from build123d import *

# Parameters (mm, degrees)
SKETCH158_R          = 1.85
PAD009_DEPTH         = 6
SKETCH159_R          = 5
PAD010_DEPTH         = 5
PAD010_DEPTH_BACK    = 6
SKETCH160_R          = 1.85
POCKET006_DEPTH      = 6.001
POCKET006_DEPTH_BACK = 5.001
POCKET007_DEPTH      = 3
SKETCH162_W          = 18
SKETCH162_H          = 8
PAD011_DEPTH         = 2
PAD011_DEPTH_BACK    = 9
PAD012_DEPTH         = 12
POCKET008_DEPTH      = 5
CHAMFER_SIZE         = 1


with BuildPart() as part:
    # Sketch158 → Pad009 (new body)
    with BuildSketch(Plane.XY):
        Polygon((-91, -102), (-91, 88), (0, 88), (0, 79), (-70, 79), (-81, 68), (-81, -64), (-70, -75), (0, -75), (0, -84), (-82, -84), (-82, -102), align=None)
        with Locations((-85, 84)):
            Circle(SKETCH158_R, mode=Mode.SUBTRACT)
        with Locations((-85, -7)):
            Circle(SKETCH158_R, mode=Mode.SUBTRACT)
        with Locations((-85, -98)):
            Circle(SKETCH158_R, mode=Mode.SUBTRACT)
        with Locations((-85, 43)):
            Circle(SKETCH158_R, mode=Mode.SUBTRACT)
        with Locations((-85, -37)):
            Circle(SKETCH158_R, mode=Mode.SUBTRACT)
    pad009 = extrude(amount=PAD009_DEPTH)

    # Mirrored: Pad009 across Sketch158 V_Axis
    add(pad009.mirror(Plane(origin=(0, 0, 0), x_dir=(0, 0, 1), z_dir=(1, 0, 0))))

    # Sketch159 → Pad010 (join, two sides)
    with BuildSketch(Plane.XY.offset(6)) as pad010_sk:
        with Locations((-79, 78)):
            Circle(SKETCH159_R)
        with Locations((-79, -76.94)):
            Circle(SKETCH159_R)
        with Locations((78.48, -76.94)):
            Circle(SKETCH159_R)
        with Locations((78.48, 55.14)):
            Circle(SKETCH159_R)
    extrude(amount=PAD010_DEPTH)
    extrude(pad010_sk.sketch, amount=-PAD010_DEPTH_BACK)

    # Sketch160 → Pocket006 (cut, two sides)
    with BuildSketch(Plane.XY.offset(6)) as pocket006_sk:
        with Locations((-79, 78)):
            Circle(SKETCH160_R)
        with Locations((-79, -76.94)):
            Circle(SKETCH160_R)
        with Locations((78.48, -76.94)):
            Circle(SKETCH160_R)
        with Locations((78.48, 55.14)):
            Circle(SKETCH160_R)
    extrude(amount=-POCKET006_DEPTH, mode=Mode.SUBTRACT)
    extrude(pocket006_sk.sketch, amount=POCKET006_DEPTH_BACK, mode=Mode.SUBTRACT)

    # Sketch161 → Pocket007 (cut)
    with BuildSketch(Plane.XY.offset(11)):
        Polygon((-75.709103, 78), (-77.354552, 80.85), (-80.645448, 80.85), (-82.290897, 78), (-80.645448, 75.15), (-77.354552, 75.15), align=None)
        Polygon((81.770897, 55.14), (80.125448, 57.99), (76.834552, 57.99), (75.189103, 55.14), (76.834552, 52.29), (80.125448, 52.29), align=None)
        Polygon((81.770897, -76.94), (80.125448, -74.09), (76.834552, -74.09), (75.189103, -76.94), (76.834552, -79.79), (80.125448, -79.79), align=None)
        Polygon((-75.709103, -76.94), (-77.354552, -74.09), (-80.645448, -74.09), (-82.290897, -76.94), (-80.645448, -79.79), (-77.354552, -79.79), align=None)
    extrude(amount=-POCKET007_DEPTH, mode=Mode.SUBTRACT)

    # Sketch162 → Pad011 (join, two sides)
    with BuildSketch(Plane(origin=(0, 88, 0), x_dir=(-1, 0, 0), z_dir=(0, 1, 0))) as pad011_sk:
        with Locations((67, 4)):
            Rectangle(SKETCH162_W, SKETCH162_H)
    extrude(amount=PAD011_DEPTH)
    extrude(pad011_sk.sketch, amount=-PAD011_DEPTH_BACK)

    # Sketch166 (on Face53 of Pad011) → Pad012 (join)
    with BuildSketch(Plane(origin=(0, 90, 0), x_dir=(-1, 0, 0), z_dir=(0, 1, 0))):
        Polygon((73, 0), (65, 0), (65, 116), (103, 116), (103, 111), (73, 111), align=None)
    extrude(amount=PAD012_DEPTH)

    # Sketch167 (on Face88 of Pad012) → Pocket008 (cut)
    with BuildSketch(Plane.XY.offset(116)):
        with BuildLine():
            ThreePointArc((-97.5, 98.5), (-100, 96), (-97.5, 93.5))
            Line((-97.5, 93.5), (-82.5, 93.5))
            ThreePointArc((-82.5, 93.5), (-80, 96), (-82.5, 98.5))
            Line((-97.5, 98.5), (-82.5, 98.5))
        make_face()
    extrude(amount=-POCKET008_DEPTH, mode=Mode.SUBTRACT)

    # Chamfer
    chamfer_edges = [part.edges().sort_by_distance(p)[0] for p in [
        (-69, 90, 8),
    ]]
    chamfer(chamfer_edges, length=CHAMFER_SIZE)


with BuildPart() as part_1:
    # Body006 placement: moved
    add(part.part.moved(Location((0, 2, 118))))


solid = part_1.part
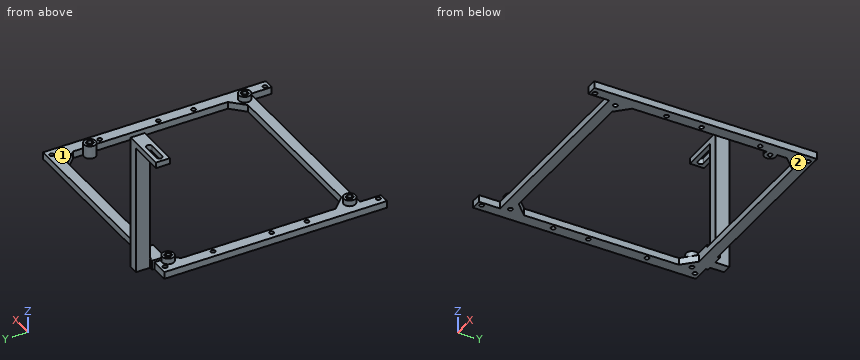
Input: part model. Units: mm. Frame: model coordinates. Face numbers are marked on the shaded views. Give positions to 0.01 mm unless a question says otherwise; leave off trailing zeros. Loops run counter-clockwise (first coordinate to the right, second up) from the corner with the lowest first, then second, coordinate; pieces in that order, holes last. Notation, with made-up numbers: (78.5, -14) -> (125.5, -14) arc R11 cw to (125.5, 3) -> close; hole circle Ø4 at (-5, -35.5). An arc over 180 degrees is marked (long way). Answer as a JSON object with one key per item and string values. Group by question number.
Item 1: Pin query (flat end, axial travel): P1, Ø6.5, axis at x = 78, y = -74, coming from the +Z side; P2, Ø0.9, axis at x = 78, z = 127.5, coming from the +Y side; P3, Ø1.5, axis at x = -78.5, z = 128, coming from the +Y side. Return the tip coordinate at first contact, or that it passes through.
Item 2: Cut plane B-B, the plane x = 21. Return the cut outline in (y, z), and give its area (3 significant figures).
Item 3: Cut plane A-A, the plane y = -15.5. Return the cut outline in (x, z).
Item 4: Cut plane C-C, the plane z = 195.5. Return the cut outline in (x, y), and give its area (3 significant figures).
Item 5: Line query: probe 1 along Y at (x, z) = (85, 120); probe 2 along X at (y, z) = (-74.94, 122.25); probe 3 along X at (y, z) = (86, 119.3). Output: solid intervals per line, ascending.
Item 6: Pull-direction query (X, two-part tool) for the marked faces 1 and 2; classes: released by +X, released by -X, zero draft, split by the parting line, or undercut.
Checks:
{
 "1": {"P1": "stops at z = 129", "P2": "stops at y = 62.14", "P3": "stops at y = 85"},
 "2": {"outline": "(-82, 118) -> (-73, 118) -> (-73, 124) -> (-82, 124) -> close; (81, 118) -> (90, 118) -> (90, 124) -> (81, 124) -> close", "area": "108 mm²"},
 "3": {"outline": "(-91, 118) -> (-81, 118) -> (-81, 124) -> (-91, 124) -> close; (81, 118) -> (91, 118) -> (91, 124) -> (81, 124) -> close"},
 "4": {"outline": "(-73, 92) -> (-65, 92) -> (-65, 104) -> (-73, 104) -> close", "area": "96.0 mm²"},
 "5": {"probe 1": "y = -100 to -97.85, -94.15 to -36.85, -33.15 to -6.85, -3.15 to 43.15, 46.85 to 84.15, 87.85 to 90", "probe 2": "x = -91 to -80.85, -77.15 to 76.63, 80.33 to 91", "probe 3": "x = -91 to -86.85, -83.15 to 83.15, 86.85 to 91"},
 "6": {"face 1": "undercut", "face 2": "zero draft"}
}
